Can you work these out from the drawing? Everything is in mm from the part's minimum corner. Round coordinates to 2 decimals unless told otherwise and drop trailing zeros. Order: outer loops, then holes, each group sorted by start corner. A loop starts at its lowest first (then second) coordinate and runs counter-clockwise, first axis right, second up. Notation, with made-up numbers: M -20.5,33 L -14.5,33 A13 cw -14.5,41 Z; hole C -25.5,-6 d5. An arc over 180 degrees is marked long. Write item = value, one per line. Start each with the question number.
Item 1: I want a section at C-C, the plane z = 4. List the corners of the cut face in (x, y) for me.
Item 2: I want a section at B-B, the plane x = 61. List the corners of the cut face in (y, z) for me.
Item 3: Please list where these lines run through material, in increasing order: L1, parallel to X at y = 27, z = 1.5; L2, parallel to Y at x = 36.5, z = 1.8; L3, parallel to Y at x = 79.5, z = 1.15.
Item 4: I want a section at A-A, the plane y = 21. List the corners of the cut face in (x, z) for me, plus the area to 3 significant figures.
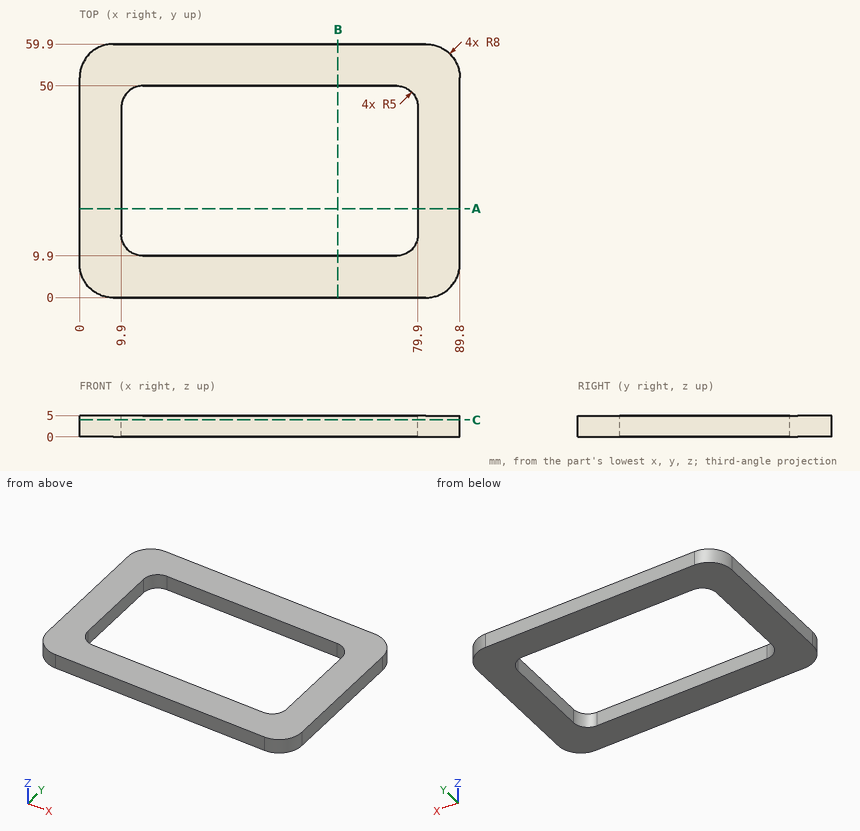
Filled in:
q1.outline = M 0,8 A8 ccw 8,0 L 81.8,0 A8 ccw 89.8,8 L 89.8,51.9 A8 ccw 81.8,59.9 L 8,59.9 A8 ccw 0,51.9 Z; hole M 9.9,14.9 A5 ccw 14.9,9.9 L 74.9,9.9 A5 ccw 79.9,14.9 L 79.9,45 A5 ccw 74.9,50 L 14.9,50 A5 ccw 9.9,45 Z
q2.outline = M 0,0 L 9.9,0 L 9.9,5 L 0,5 Z; M 50,0 L 59.9,0 L 59.9,5 L 50,5 Z
q3.L1 = 0 to 9.9, 79.9 to 89.8
q3.L2 = 0 to 9.9, 50 to 59.9
q3.L3 = 0 to 12.94, 46.96 to 59.9
q4.outline = M 0,0 L 9.9,0 L 9.9,5 L 0,5 Z; M 79.9,0 L 89.8,0 L 89.8,5 L 79.9,5 Z
q4.area = 99.0 mm^2
